For this review, take the finished solid that the model builds, in its own axes (mm). A direction names the side the tool comes from. Coordinates: 2 decimals unless noted, no trailing zeros. Order: outer loops, then holes, each group sorted by start corner. A loop starts at its lowest first (then second) coordinate and runs counter-clockwise, first axis right, second up. Notation, with made-up numbers: (54.5, -5) -> (94.5, -5) arc R9 cw to (94.5, 7) -> close; hole circle Ø7 at (-25, 40). An arc over 180 degrees is marked (long way). Return JSON: item names as keys, results as strings. Group by question number.
Item 1: Insertion check: pin 1 (10 mm diameter, centred on x = -2, y = 9.5, fed in from +Z); pin 2 (3.5 mm diameter, centred on x = 0.5, z = -50, fed in from +Y); pin 3 (0.9 mm diameter, centred on y = 0, z = -35.5, fed in from +X) (3 decimals); pin 4 (2.5 mm diameter, centred on x = 0.5, z = -52, fed in from -Y). Each pin has a flat end and moves straight along its axis. Give the tip position at first contact, or say it passes through.
Item 2: For line 1 along Y through (x, z) = (0, -73) (3 decimals); line 2 along X through (y, z) = (6.25, -9); line 3 along Y through (x, z) = (5.25, -66), list the stretches that pass through material, from the lowest coordinate up.
Item 3: Machinability: for faces 4 (the cylindrical face through (-11.94, -11.91, -49.3)), 5 (the flat face through (-5, -10.36, -49)), which of the approach directions +Z, -Z, +X, -X, +Y, -Y give a long, thin tool a straight path to every point of the face, cutting with its end or side? Answer none if there is none.
Item 4: Draft analysis for pull direction Y (two halves, no side actions). For faces 1 (the flat face through (0, 3, 0)), 2 (the flat face through (7, -12.5, -49)), 3 (the cylindrical face through (11.45, -3.25, -49.3)), state which applies: +Y half, -Y half, draft (parallel to the pull), parting line (faces both ways), or undercut.
Item 5: Take a section at B-B (y = 11.43). Write out the cut boundary in (x, z).
Item 6: Take a section at A-A (x = 0). Write out the cut boundary in (y, z) (3 decimals), then the cut area to 3 significant figures.
Autodesk Inventor part; units mm, degrees
ref_plane "YZ Plane" through (0, 0, 0) normal (1, 0, 0) x (0, 1, 0)
ref_plane "XZ Plane" through (0, 0, 0) normal (0, 1, 0) x (-1, 0, 0)
ref_plane "XY Plane" through (0, 0, 0) normal (0, 0, 1) x (1, 0, 0)
sketch "Sketch1" plane through (0, 0, 0) normal (0, 0, 1) x (1, 0, 0)
  circle A0 centre (0, 0) radius 2.5
  arc A1 (-8.6363, 7.1116) -> (-10.36, 6.3969) centre (-9.35, 6.3969) ccw
  line L0 (-8.6363, 7.1116) -> (-5.4322, 3.9121)
  arc A2 (-4.455, 1.5554) -> (-5.4322, 3.9121) centre (-7.7855, 1.5554) ccw
  line L1 (-4.455, 1.5554) -> (-4.455, -1.5554)
  arc A3 (-5.4322, -3.9121) -> (-4.455, -1.5554) centre (-7.7855, -1.5554) ccw
  line L2 (-5.4322, -3.9121) -> (-8.6363, -7.1116)
  arc A4 (-10.36, -6.3969) -> (-8.6363, -7.1116) centre (-9.35, -6.3969) ccw
  line L3 (-10.36, -6.3969) -> (-10.36, -4.32)
  arc A5 (-10.36, -4.32) -> (-12.5, -4.32) centre (-11.43, -4.32) ccw
  line L4 (-12.5, -4.32) -> (-12.5, -10.5371)
  arc A6 (-12.5, -10.5371) -> (-10.5371, -12.5) centre (-10.5371, -10.5371) ccw
  line L5 (-10.5371, -12.5) -> (-4.3879, -12.5)
  arc A7 (-4.3879, -12.5) -> (-4.3879, -10.36) centre (-4.3879, -11.43) ccw
  line L6 (-4.3879, -10.36) -> (-6.42, -10.36)
  arc A8 (-7.1337, -8.6353) -> (-6.42, -10.36) centre (-6.42, -9.35) ccw
  line L7 (-7.1337, -8.6353) -> (-3.7953, -5.3018)
  arc A9 (-1.5554, -4.375) -> (-3.7953, -5.3018) centre (-1.5554, -7.545) ccw
  line L8 (-1.5554, -4.375) -> (1.5554, -4.375)
  arc A10 (3.7953, -5.3018) -> (1.5554, -4.375) centre (1.5554, -7.545) ccw
  line L9 (3.7953, -5.3018) -> (7.1337, -8.6353)
  arc A11 (6.42, -10.36) -> (7.1337, -8.6353) centre (6.42, -9.35) ccw
  line L10 (6.42, -10.36) -> (4.3879, -10.36)
  arc A12 (4.3879, -10.36) -> (4.3879, -12.5) centre (4.3879, -11.43) ccw
  line L11 (4.3879, -12.5) -> (10.5371, -12.5)
  arc A13 (10.5371, -12.5) -> (12.5, -10.5371) centre (10.5371, -10.5371) ccw
  line L12 (12.5, -10.5371) -> (12.5, -4.32)
  arc A14 (12.5, -4.32) -> (10.36, -4.32) centre (11.43, -4.32) ccw
  line L13 (10.36, -4.32) -> (10.36, -6.3969)
  arc A15 (8.6363, -7.1116) -> (10.36, -6.3969) centre (9.35, -6.3969) ccw
  line L14 (8.6363, -7.1116) -> (5.4322, -3.9121)
  arc A16 (4.455, -1.5554) -> (5.4322, -3.9121) centre (7.7855, -1.5554) ccw
  line L15 (4.455, -1.5554) -> (4.455, 1.5554)
  arc A17 (5.4322, 3.9121) -> (4.455, 1.5554) centre (7.7855, 1.5554) ccw
  line L16 (5.4322, 3.9121) -> (8.6363, 7.1116)
  arc A18 (10.36, 6.3969) -> (8.6363, 7.1116) centre (9.35, 6.3969) ccw
  line L17 (10.36, 6.3969) -> (10.36, 4.32)
  arc A19 (10.36, 4.32) -> (12.5, 4.32) centre (11.43, 4.32) ccw
  line L18 (12.5, 4.32) -> (12.5, 10.5371)
  arc A20 (12.5, 10.5371) -> (10.5371, 12.5) centre (10.5371, 10.5371) ccw
  line L19 (10.5371, 12.5) -> (4.32, 12.5)
  arc A21 (4.32, 12.5) -> (4.32, 10.36) centre (4.32, 11.43) ccw
  line L20 (4.32, 10.36) -> (6.42, 10.36)
  arc A22 (7.1337, 8.6353) -> (6.42, 10.36) centre (6.42, 9.35) ccw
  line L21 (7.1337, 8.6353) -> (3.7953, 5.3018)
  arc A23 (1.5554, 4.375) -> (3.7953, 5.3018) centre (1.5554, 7.545) ccw
  line L22 (1.5554, 4.375) -> (-1.5554, 4.375)
  arc A24 (-3.7953, 5.3018) -> (-1.5554, 4.375) centre (-1.5554, 7.545) ccw
  line L23 (-3.7953, 5.3018) -> (-7.1337, 8.6353)
  arc A25 (-6.42, 10.36) -> (-7.1337, 8.6353) centre (-6.42, 9.35) ccw
  line L24 (-6.42, 10.36) -> (-4.32, 10.36)
  arc A26 (-4.32, 10.36) -> (-4.32, 12.5) centre (-4.32, 11.43) ccw
  line L25 (-4.32, 12.5) -> (-10.5371, 12.5)
  arc A27 (-10.5371, 12.5) -> (-12.5, 10.5371) centre (-10.5371, 10.5371) ccw
  line L26 (-12.5, 10.5371) -> (-12.5, 4.32)
  arc A28 (-12.5, 4.32) -> (-10.36, 4.32) centre (-11.43, 4.32) ccw
  line L27 (-10.36, 4.32) -> (-10.36, 6.3969)
extrude "Extrusion1" add sketch "Sketch1" against normal blind 100
properties part number "25-2525"
Findings below:
{
 "1": {"pin 1": "stops at z = 0", "pin 2": "stops at y = 4.45", "pin 3": "stops at x = 4.455", "pin 4": "stops at y = -4.38"},
 "2": {"line 1": "y = -4.375 to -2.5, 2.5 to 4.375", "line 2": "x = -12.5 to -10.36, -7.77 to -4.74, 4.74 to 7.77, 10.36 to 12.5", "line 3": "y = -12.5 to -10.36, -6.75 to -3.71, 3.71 to 6.75, 10.36 to 12.5"},
 "3": {"face 4": "+Z, -Z, -X, -Y", "face 5": "+Z, -Z"},
 "4": {"face 1": "draft", "face 2": "-Y half", "face 3": "undercut"},
 "5": {"outline": "(-12.29, -100) -> (-3.25, -100) -> (-3.25, 0) -> (-12.29, 0) -> close; (3.25, -100) -> (12.29, -100) -> (12.29, 0) -> (3.25, 0) -> close"},
 "6": {"outline": "(-4.375, -100) -> (-2.5, -100) -> (-2.5, 0) -> (-4.375, 0) -> close; (2.5, -100) -> (4.375, -100) -> (4.375, 0) -> (2.5, 0) -> close", "area": "375 mm2"}
}
